```python
from build123d import *

# Parameters (mm, degrees)
SKETCH_W        = 19.8
SKETCH_H        = 28.8
PAD_DEPTH       = 6.4
SKETCH001_W     = 17.4
SKETCH001_H     = 26.4
POCKET_DEPTH    = 1.9
SKETCH002_W     = 15
SKETCH002_H     = 24
POCKET001_DEPTH = 2.5
SKETCH004_R     = 1
POCKET002_DEPTH = 6.5
CHAMFER_SIZE    = 0.5
CHAMFER001_SIZE = 0.5
CHAMFER002_SIZE = 0.5
CHAMFER003_SIZE = 0.5
FILLET_R        = 1.4
FILLET001_R     = 0.5
FILLET002_R     = 2.6
FILLET003_R     = 0.5
FILLET004_R     = 0.5
FILLET005_R     = 0.5
FILLET006_R     = 1.2
FILLET007_R     = 1.2
FILLET008_R     = 1.2
FILLET009_R     = 2.6
FILLET010_R     = 2.6
FILLET011_R     = 2.6
SKETCH005_R     = 2
POCKET003_DEPTH = 1.5
CHAMFER004_SIZE = 0.8


with BuildPart() as part:
    # Sketch → Pad (new body)
    with BuildSketch(Plane.XY):
        Rectangle(SKETCH_W, SKETCH_H)
    extrude(amount=PAD_DEPTH)

    # Sketch001 (on Face6 of Pad) → Pocket (cut)
    with BuildSketch(Plane.XY.offset(6.4)):
        Rectangle(SKETCH001_W, SKETCH001_H)
    extrude(amount=-POCKET_DEPTH, mode=Mode.SUBTRACT)

    # Sketch002 (on Face11 of Pocket) → Pocket001 (cut)
    with BuildSketch(Plane.XY.offset(4.5)):
        Rectangle(SKETCH002_W, SKETCH002_H)
    extrude(amount=-POCKET001_DEPTH, mode=Mode.SUBTRACT)

    # Sketch004 → Pocket002 (cut)
    with BuildSketch(Plane.XY.offset(6.5)):
        with Locations((4.5, 2.5)):
            Circle(SKETCH004_R)
    extrude(amount=-POCKET002_DEPTH, mode=Mode.SUBTRACT)

    # Chamfer
    chamfer_edges = [part.edges().sort_by_distance(p)[0] for p in [
        (0, 12, 2),
    ]]
    chamfer(chamfer_edges, length=CHAMFER_SIZE)

    # Chamfer001
    chamfer001_edges = [part.edges().sort_by_distance(p)[0] for p in [
        (-7.5, -0.25, 2),
    ]]
    chamfer(chamfer001_edges, length=CHAMFER001_SIZE)

    # Chamfer002
    chamfer002_edges = [part.edges().sort_by_distance(p)[0] for p in [
        (7.5, -0.25, 2),
    ]]
    chamfer(chamfer002_edges, length=CHAMFER002_SIZE)

    # Chamfer003
    chamfer003_edges = [part.edges().sort_by_distance(p)[0] for p in [
        (0, -12, 2),
    ]]
    chamfer(chamfer003_edges, length=CHAMFER003_SIZE)

    # Fillet
    fillet_edges = [part.edges().sort_by_distance(p)[0] for p in [
        (-8.7, 13.2, 5.45),
    ]]
    fillet(fillet_edges, radius=FILLET_R)

    # Fillet001
    fillet001_edges = [part.edges().sort_by_distance(p)[0] for p in [
        (-7.5, 12, 3.5),
    ]]
    fillet(fillet001_edges, radius=FILLET001_R)

    # Fillet002
    fillet002_edges = [part.edges().sort_by_distance(p)[0] for p in [
        (-9.9, 14.4, 3.2),
    ]]
    fillet(fillet002_edges, radius=FILLET002_R)

    # Fillet003
    fillet003_edges = [part.edges().sort_by_distance(p)[0] for p in [
        (7.5, 12, 3.5),
    ]]
    fillet(fillet003_edges, radius=FILLET003_R)

    # Fillet004
    fillet004_edges = [part.edges().sort_by_distance(p)[0] for p in [
        (-7.5, -12, 3.5),
    ]]
    fillet(fillet004_edges, radius=FILLET004_R)

    # Fillet005
    fillet005_edges = [part.edges().sort_by_distance(p)[0] for p in [
        (7.5, -12, 3.5),
    ]]
    fillet(fillet005_edges, radius=FILLET005_R)

    # Fillet006
    fillet006_edges = [part.edges().sort_by_distance(p)[0] for p in [
        (8.7, -13.2, 5.45),
    ]]
    fillet(fillet006_edges, radius=FILLET006_R)

    # Fillet007
    fillet007_edges = [part.edges().sort_by_distance(p)[0] for p in [
        (-8.7, -13.2, 5.45),
    ]]
    fillet(fillet007_edges, radius=FILLET007_R)

    # Fillet008
    fillet008_edges = [part.edges().sort_by_distance(p)[0] for p in [
        (8.7, 13.2, 5.45),
    ]]
    fillet(fillet008_edges, radius=FILLET008_R)

    # Fillet009
    fillet009_edges = [part.edges().sort_by_distance(p)[0] for p in [
        (9.9, 14.4, 3.2),
    ]]
    fillet(fillet009_edges, radius=FILLET009_R)

    # Fillet010
    fillet010_edges = [part.edges().sort_by_distance(p)[0] for p in [
        (9.9, -14.4, 3.2),
    ]]
    fillet(fillet010_edges, radius=FILLET010_R)

    # Fillet011
    fillet011_edges = [part.edges().sort_by_distance(p)[0] for p in [
        (-9.9, -14.4, 3.2),
    ]]
    fillet(fillet011_edges, radius=FILLET011_R)

    # Sketch005 (on Face18 of Fillet011) → Pocket003 (cut)
    with BuildSketch(Plane(origin=(0, 0, 0), x_dir=(1, 0, 0), z_dir=(0, 0, -1))):
        with Locations((4.5, -2.5)):
            Circle(SKETCH005_R)
    extrude(amount=-POCKET003_DEPTH, mode=Mode.SUBTRACT)

    # Chamfer004
    chamfer004_edges = [part.edges().sort_by_distance(p)[0] for p in [
        (2.5, 2.5, 1.5),
    ]]
    chamfer(chamfer004_edges, length=CHAMFER004_SIZE)


solid = part.part
```
Check sheet for the modelled part. Datum: model origin and axes. Units: mm. A direction names the side the tool comes from. Round coordinates to 2 decimals unless told otherwise and drop trailing zeros. Loops run counter-clockwise (first coordinate to the right, second up) from the corner with the lowest first, then second, coordinate; pieces in that order, holes last. Notation, with made-up numbers: (27, 48.5) - (82, 48.5) arc R20 ccw to (82, 76.5) - close; hole circle Ø11 at (19, 89). An arc over 180 degrees is marked (long way). Answer as a JSON object with one key per item and string values. Group by question number.
Q1. Sectioned sample at C-C, the plane z = 3.5. Enter the section's corners in (x, y), plus the area to 3 significant figures.
Q2. Sectioned sample at A-A, the plane y = 2.5. Enter the section's corners in (x, z), plus the area to 4 significant figures.
Q3. Gauge pin test, flat ends, axial feed: P1, Ø6.5, axis at x = 4.5, y = 2.5, coming from the +Z side; P2, Ø1, axis at x = 2, y = 4.5, coming from the +Z side; P3, Ø2.5, axis at x = 4, y = 2.5, coming from the -Z side. Record the tip position at first contact, or that the pin passes through.
Q4. Set-up check for faces 4 (the face through (-9, 0, 6.4)), 5 (the face through (0, 0, 2)): record each of +Z, -Z, +X, -X, +Y, -Y from which the full face is reachable in a straight line by a thin tool's end or side.
Q5. Sectioned sample at B-B, the plane x = 4.5. Enter the section's corners in (y, z), plus the area to 4 significant figures.
Q6. Sectioned sample at D-D, the plane y = -2.75. Enter the section's corners in (x, z).
Q7. Scan lines: line 1 along Y through (x, z) = (4.5, 1.9); line 2 along X through (y, z) = (-4.5, 5.5); line 3 along Y through (x, z) = (-2.5, 2.5). Record each from-to range of solid material in increasing order. Write a range as [from, to].
Q8. Mould release check, pull along X, two halves, no side actions. Record for faces 1 (the face through (-9.9, 0, 3)), 2 (the face through (9.118, 13.659, 3.245)), 3 (the face through (2.502, 2.412, 0.345)): released by +X, released by -X, zero draft, split by the parting line, or undercut.
Solution:
{
 "1": {"outline": "(-9.9, -11.8) arc R2.6 ccw to (-7.3, -14.4) - (7.3, -14.4) arc R2.6 ccw to (9.9, -11.8) - (9.9, 11.8) arc R2.6 ccw to (7.3, 14.4) - (-7.3, 14.4) arc R2.6 ccw to (-9.9, 11.8) - close; hole (-7.5, -11.5) arc R0.5 ccw to (-7, -12) - (7, -12) arc R0.5 ccw to (7.5, -11.5) - (7.5, 11.5) arc R0.5 ccw to (7, 12) - (-7, 12) arc R0.5 ccw to (-7.5, 11.5) - close", "area": "205 mm²"},
 "2": {"outline": "(-9.9, 0) - (2.5, 0) - (2.5, 0.7) - (3.3, 1.5) - (3.5, 1.5) - (3.5, 2) - (-7, 2) - (-7.5, 2.5) - (-7.5, 4.5) - (-8.7, 4.5) - (-8.7, 6.4) - (-9.9, 6.4) - close; (5.5, 1.5) - (5.7, 1.5) - (6.5, 0.7) - (6.5, 0) - (9.9, 0) - (9.9, 6.4) - (8.7, 6.4) - (8.7, 4.5) - (7.5, 4.5) - (7.5, 2.5) - (7, 2) - (5.5, 2) - close", "area": "50.05 mm²"},
 "3": {"P1": "stops at z = 4.5", "P2": "stops at z = 2", "P3": "stops at z = 0.95"},
 "4": {"face 4": "+Z, +X, -X, +Y, -Y", "face 5": "+Z"},
 "5": {"outline": "(-14.4, 0) - (0.5, 0) - (0.5, 0.7) - (1.3, 1.5) - (1.5, 1.5) - (1.5, 2) - (-11.5, 2) - (-12, 2.5) - (-12, 4.5) - (-13.2, 4.5) - (-13.2, 6.4) - (-14.4, 6.4) - close; (3.5, 1.5) - (3.7, 1.5) - (4.5, 0.7) - (4.5, 0) - (14.4, 0) - (14.4, 6.4) - (13.2, 6.4) - (13.2, 4.5) - (12, 4.5) - (12, 2.5) - (11.5, 2) - (3.5, 2) - close", "area": "68.05 mm²"},
 "6": {"outline": "(-9.9, 0) - (9.9, 0) - (9.9, 6.4) - (8.7, 6.4) - (8.7, 4.5) - (7.5, 4.5) - (7.5, 2.5) - (7, 2) - (-7, 2) - (-7.5, 2.5) - (-7.5, 4.5) - (-8.7, 4.5) - (-8.7, 6.4) - (-9.9, 6.4) - close"},
 "7": {"line 1": "y = [-14.4, 1.5], [3.5, 14.4]", "line 2": "x = [-9.9, -8.7], [8.7, 9.9]", "line 3": "y = [-14.4, -12], [12, 14.4]"},
 "8": {"face 1": "released by -X", "face 2": "released by +X", "face 3": "undercut"}
}
